from build123d import *

# Parameters (mm, degrees)
SKETCH006_W            = 40
SKETCH006_H            = 113.480256
PAD001_DEPTH           = 2
FILLET_R               = 5
FILLET001_R            = 5
FILLET002_R            = 5
FILLET003_R            = 5
POCKET003_DEPTH        = 242.68144
LINEARPATTERN001_COUNT = 6
LINEARPATTERN001_PITCH = 18


with BuildPart() as part:
    # Sketch006 → Pad001 (new body)
    with BuildSketch(Plane.XY.offset(40)):
        Rectangle(SKETCH006_W, SKETCH006_H)
    extrude(amount=PAD001_DEPTH)

    # Fillet
    fillet_edges = [part.edges().sort_by_distance(p)[0] for p in [
        (20, 56.740128, 41),
    ]]
    fillet(fillet_edges, radius=FILLET_R)

    # Fillet001
    fillet001_edges = [part.edges().sort_by_distance(p)[0] for p in [
        (-20, 56.740128, 41),
    ]]
    fillet(fillet001_edges, radius=FILLET001_R)

    # Fillet002
    fillet002_edges = [part.edges().sort_by_distance(p)[0] for p in [
        (-20, -56.740128, 41),
    ]]
    fillet(fillet002_edges, radius=FILLET002_R)

    # Fillet003
    fillet003_edges = [part.edges().sort_by_distance(p)[0] for p in [
        (20, -56.740128, 41),
    ]]
    fillet(fillet003_edges, radius=FILLET003_R)

    # Sketch007 → Pocket003 (cut, through all)
    with BuildSketch(Plane.XY.offset(42)):
        with BuildLine():
            ThreePointArc((-15.079723, 48.539704), (-16.741783, 46.877644), (-15.079723, 45.215584))
            Line((-15.079723, 45.215584), (15.079723, 45.215584))
            ThreePointArc((15.079723, 45.215584), (16.741783, 46.877644), (15.079723, 48.539704))
            Line((-15.079723, 48.539704), (15.079723, 48.539704))
        make_face()
    pocket003 = extrude(amount=-POCKET003_DEPTH, mode=Mode.SUBTRACT)

    # LinearPattern001: Pocket003 ×6
    with Locations(*[(0, -i * LINEARPATTERN001_PITCH, 0) for i in range(1, LINEARPATTERN001_COUNT)]):
        add(pocket003, mode=Mode.SUBTRACT)


solid = part.part
Could you check a few things on this model? Use its own coordinates, in mm. A direction names the side the tool comes from. Round coordinates to 2 decimals unless told otherwise and drop trailing zeros. Order: outer loops, then holes, each group sorted by start corner. A loop starts at its lowest first (then second) coordinate and runs counter-clockwise, first axis right, second up.
Q1. Imagine slicing it at B-B, the plane z = 41.25. State how many separate pieces and enclosed holes the cut face has, then the cut area to 3 significant figures.
Geometry says:
separate pieces: 1
enclosed holes: 6
area: 3,860 mm2
Q2. Which directions (+Z, -Z, +X, -X, +Y, -Y) give clear straight access to the entire face, cutting with the end or side of a thin tool? Please do faces 1 (the face through (0, 30.54, 41)), 2 (the face through (0, 56.74, 41)).
Geometry says:
face 1: +Z, -Z
face 2: +Z, -Z, +X, -X, +Y
Q3. Thinking about a two-plate mould opening in X: for faces 3 (the face through (18.57, 55.24, 41.01)), 4 (the face through (-16.74, 10.91, 41.01)), 5 (the face through (0, 1, 40)), 6 (the face through (-18.57, -55.24, 41.01)), which applies, released by +X, released by -X, zero draft, split by the parting line, or undercut?
Geometry says:
face 3: released by +X
face 4: undercut
face 5: zero draft
face 6: released by -X
Q4. Imagine slicing it at A-A, the plane x = -3. List the corners of the cut face in (y, z) for me, then the cut area to 3 significant figures.
Geometry says:
outline: (-56.74, 40) - (-44.78, 40) - (-44.78, 42) - (-56.74, 42) - close; (-41.46, 40) - (-26.78, 40) - (-26.78, 42) - (-41.46, 42) - close; (-23.46, 40) - (-8.78, 40) - (-8.78, 42) - (-23.46, 42) - close; (-5.46, 40) - (9.22, 40) - (9.22, 42) - (-5.46, 42) - close; (12.54, 40) - (27.22, 40) - (27.22, 42) - (12.54, 42) - close; (30.54, 40) - (45.22, 40) - (45.22, 42) - (30.54, 42) - close; (48.54, 40) - (56.74, 40) - (56.74, 42) - (48.54, 42) - close
area: 187 mm2
Q5. Please list where these lines run through material, in increasing order: probe 1 along X at (y, z) = (27.5, 41.9); probe 2 along X at (y, z) = (30, 40.8); probe 3 along Y at (x, z) = (18, 41.3).
Geometry says:
probe 1: x = -20 to -16.01, 16.01 to 20
probe 2: x = -20 to -16.31, 16.31 to 20
probe 3: y = -55.74 to 55.74
